Can you work these out from the model? Positions are in its coordinate system, mm. A direction names the side the tool comes from. Round coordinates to 2 decimals unless told otherwise and drop trailing zeros. Use one line per item in the form item = value. Start each with the question number.
```python
from build123d import *
from build123d.topology import SkipClean

# Parameters (mm, degrees)
BOSS_EXTRUDE1_DEPTH = 45
SKETCH4_R           = 2.375
BOSS_EXTRUDE3_DEPTH = 2
FILLET1_R           = 0.5
BOSS_EXTRUDE5_START = 2
SKETCH6_R           = 2.375
BOSS_EXTRUDE5_DEPTH = 2
FILLET2_R           = 1


with BuildPart() as part:
    # Sketch2 → Boss-Extrude1 (new body)
    with BuildSketch(Plane(origin=(0, 0, 0), x_dir=(1, 0, 0), z_dir=(0, 1, 0))):
        with BuildLine():
            Line((3.775215965, -0.978645895), (2.300774305, -0.58912019))
            ThreePointArc((2.300774305, -0.58912019), (2.374963211, 0.013219106), (2.294073837, 0.614695232))
            Line((2.294073837, 0.614695232), (3.742962577, 1.0029238))
            ThreePointArc((3.742962577, 1.0029238), (3.356294138, 1.936727823), (2.741299364, 2.73877761))
            Line((2.741299364, 2.73877761), (1.680151223, 1.678605632))
            ThreePointArc((1.680151223, 1.678605632), (1.187973207, 2.056537055), (0.614695232, 2.294073837))
            Line((0.614695232, 2.294073837), (1.0029238, 3.742962577))
            ThreePointArc((1.0029238, 3.742962577), (0, 3.875), (-1.0029238, 3.742962577))
            Line((-1.0029238, 3.742962577), (-0.614695232, 2.294073837))
            ThreePointArc((-0.614695232, 2.294073837), (-1.1875, 2.056810334), (-1.679378605, 1.679378605))
            Line((-1.679378605, 1.679378605), (-2.740038777, 2.740038777))
            ThreePointArc((-2.740038777, 2.740038777), (-3.35584844, 1.9375), (-3.742962577, 1.0029238))
            Line((-3.742962577, 1.0029238), (-2.294073837, 0.614695232))
            ThreePointArc((-2.294073837, 0.614695232), (-2.375, 0), (-2.294073837, -0.614695232))
            Line((-2.294073837, -0.614695232), (-3.742962577, -1.0029238))
            ThreePointArc((-3.742962577, -1.0029238), (-3.35584844, -1.9375), (-2.740038777, -2.740038777))
            Line((-2.740038777, -2.740038777), (-1.679378605, -1.679378605))
            ThreePointArc((-1.679378605, -1.679378605), (-1.1875, -2.056810334), (-0.614695232, -2.294073837))
            Line((-0.614695232, -2.294073837), (-1.0029238, -3.742962577))
            ThreePointArc((-1.0029238, -3.742962577), (0.033967076, -3.874851125), (1.068386506, -3.724805401))
            Line((1.068386506, -3.724805401), (0.681359786, -2.275164575))
            ThreePointArc((0.681359786, -2.275164575), (1.238849907, -2.026296106), (1.714477211, -1.643530618))
            Line((1.714477211, -1.643530618), (2.767163136, -2.698133353))
            ThreePointArc((2.767163136, -2.698133353), (3.500652231, -1.972912562), (3.775215965, -0.978645895))
        make_face()
        Polygon((0.085836926, -0.044584082), (0, 0), (0.073933818, 0), (0.104207494, -0.030328801), (0.080162685, -0.023330742), align=None, mode=Mode.SUBTRACT)
    extrude(amount=BOSS_EXTRUDE1_DEPTH)

    # Sketch4 → Boss-Extrude3 (add)
    with BuildSketch(Plane(origin=(0, 45, 0), x_dir=(1, 0, 0), z_dir=(0, 1, 0))):
        with Locations(Location((0, 0, 0), (0, 0, 75))):
            Circle(SKETCH4_R)
    extrude(amount=BOSS_EXTRUDE3_DEPTH)

    # Fillet1
    # the kernel refuses this fillet: 0.5 mm, written as the material it adds along each edge
    with BuildSketch(Plane(origin=(-2.294073837, 0, 0.614695232), x_dir=(-0.1735157400494046, 0, -0.9848310961556339), z_dir=(0, 1, 0)), Plane(origin=(-1.679378605, 0, -1.679378605), x_dir=(0.7661308776829403, 0, -0.6426845869170722), z_dir=(0, 1, 0)), Plane(origin=(0.614695232, 0, -2.294073837), x_dir=(0.939646617732385, 0, 0.3421465092384974), z_dir=(0, 1, 0)), Plane(origin=(2.294073837, 0, -0.614695232), x_dir=(0.1735157400495284, 0, 0.9848310961556122), z_dir=(0, 1, 0)), Plane(origin=(-0.614695232, 0, 2.294073837), x_dir=(-0.9396466177323688, 0, -0.3421465092385419), z_dir=(0, 1, 0))) as fillet1_piece_1:
        with BuildLine():
            CenterArc((0.458270974, 0.498091484), FILLET1_R, 185.007705084, 79.984589832)
            Line((-0.03982051, 0.45444663), (0, 0))
            ThreePointArc((0, 0), (0.20731306, 0.00906545), (0.414626119, 0))
        make_face()
    extrude(amount=45)
    with BuildSketch(Plane(origin=(-2.294073837, 0, -0.614695232), x_dir=(-0.17351574004940104, 0, 0.9848310961556345), z_dir=(0, 1, 0)), Plane(origin=(-0.614695232, 0, -2.294073837), x_dir=(-0.9396466177323672, 0, 0.3421465092385461), z_dir=(0, 1, 0)), Plane(origin=(1.680151223, 0, -1.678605632), x_dir=(-0.7658350540129166, 0, -0.643037067395833), z_dir=(0, 1, 0))) as fillet1_piece_2:
        with BuildLine():
            CenterArc((0.458270974, -0.498091484), FILLET1_R, 95.007705084, 79.984589832)
            Line((-0.03982051, -0.45444663), (0, 0))
            ThreePointArc((0, 0), (0.20731306, -0.00906545), (0.414626119, 0))
        make_face()
    extrude(amount=45)
    with BuildSketch(Plane(origin=(2.300774305, 0, 0.58912019), x_dir=(0.9668296370387235, 0, 0.2554221073900419), z_dir=(0, 1, 0))) as fillet1_piece_3:
        with BuildLine():
            CenterArc((0.453002414, 0.5), FILLET1_R, 190.38170854, 79.61829146)
            ThreePointArc((-0.038812111, 0.409897433), (-0.010506812, 0.205791362), (0, 0))
            Line((0, 0), (0.453002414, 0))
        make_face()
    extrude(amount=45)
    with BuildSketch(Plane(origin=(1.714477211, 0, 1.643530618), x_dir=(0.7064632978713469, 0, 0.7077496794494086), z_dir=(0, 1, 0))) as fillet1_piece_4:
        with BuildLine():
            CenterArc((0.465508471, -0.5), FILLET1_R, 90, 81.041880237)
            ThreePointArc((-0.02839274, -0.422143763), (-0.00477723, -0.211705398), (0, 0))
            Line((0, 0), (0.465508471, 0))
        make_face()
    extrude(amount=45)
    with BuildSketch(Plane(origin=(0.681359786, 0, 2.275164575), x_dir=(0.25794627414893684, 0, 0.966159262053975), z_dir=(0, 1, 0))) as fillet1_piece_5:
        with BuildLine():
            CenterArc((0.443713653, 0.5), FILLET1_R, 191.464392376, 78.535607624)
            ThreePointArc((-0.046310555, 0.400620549), (-0.014636445, 0.201295026), (0, 0))
            Line((0, 0), (0.443713653, 0))
        make_face()
    extrude(amount=45)
    with BuildSketch(Plane(origin=(-1.679378605, 0, 1.679378605), x_dir=(-0.7071067811865471, 0, 0.707106781186548), z_dir=(0, 1, 0))) as fillet1_piece_6:
        with BuildLine():
            CenterArc((0.456187913, 0.5), FILLET1_R, 190.015410168, 79.984589832)
            ThreePointArc((-0.036192593, 0.413043478), (-0.00906545, 0.20731306), (0, 0))
            Line((0, 0), (0.456187913, 0))
        make_face()
    extrude(amount=45)
    # the kernel refuses this fillet: 0.5 mm, written as the material it takes off along each edge
    with BuildSketch(Plane(origin=(-2.740038777, -1.439160897, 2.740038777), x_dir=(-0.6526300069150477, 0, -0.7576767609436524), z_dir=(0, 1, 0)), Plane(origin=(-3.742962577, -1.439160897, -1.0029238), x_dir=(0.3298523193767966, 0, -0.9440325457322686), z_dir=(0, 1, 0)), Plane(origin=(2.741299364, -1.439160897, -2.73877761), x_dir=(0.652281279601926, 0, 0.7579769998363237), z_dir=(0, 1, 0))) as fillet1_2_piece_1:
        with BuildLine():
            CenterArc((0.538524723, -0.49861874), FILLET1_R, 85.740187873, 98.519624254)
            Line((0.039905983, -0.535758376), (0, 0))
            ThreePointArc((0, 0), (0.287832179, 0.010704768), (0.575664359, 0))
        make_face()
    extrude(amount=47.878321794, mode=Mode.SUBTRACT)
    with BuildSketch(Plane(origin=(-3.742962577, -1.439160897, 1.0029238), x_dir=(0.9659258262890679, 0, -0.2588190451025218), z_dir=(0, 1, 0)), Plane(origin=(-2.740038777, -1.439160897, -2.740038777), x_dir=(0.7071067811865476, 0, 0.7071067811865476), z_dir=(0, 1, 0)), Plane(origin=(3.742962577, -1.439160897, -1.0029238), x_dir=(-0.9659258262890681, 0, 0.25881904510252185), z_dir=(0, 1, 0)), Plane(origin=(-1.0029238, -1.439160897, 3.742962577), x_dir=(0.2588190451025216, 0, -0.9659258262890681), z_dir=(0, 1, 0))) as fillet1_2_piece_2:
        with BuildLine():
            CenterArc((0.537242519, -0.5), FILLET1_R, 90, 98.519624254)
            ThreePointArc((0.04275993, -0.574074074), (0.010704768, -0.287832179), (0, 0))
            Line((0, 0), (0.537242519, 0))
        make_face()
    extrude(amount=47.878321794, mode=Mode.SUBTRACT)
    with BuildSketch(Plane(origin=(-1.0029238, -1.439160897, -3.742962577), x_dir=(0.25881904510252174, 0, 0.965925826289068), z_dir=(0, 1, 0))) as fillet1_2_piece_3:
        with BuildLine():
            CenterArc((0.537242519, 0.5), FILLET1_R, 171.480375746, 98.519624254)
            ThreePointArc((0.04275993, 0.574074074), (0.010704768, 0.287832179), (0, 0))
            Line((0, 0), (0.537242519, 0))
        make_face()
    extrude(amount=47.878321794, mode=Mode.SUBTRACT)
    with BuildSketch(Plane(origin=(1.0029238, -1.439160897, -3.742962577), x_dir=(-0.9824823262918377, 0, -0.1863557847886099), z_dir=(0, 1, 0))) as fillet1_2_piece_4:
        with BuildLine():
            CenterArc((0.538524723, 0.49861874), FILLET1_R, 175.740187873, 98.519624254)
            Line((0.039905983, 0.535758376), (0, 0))
            ThreePointArc((0, 0), (0.287832179, -0.010704768), (0.575664359, 0))
        make_face()
    extrude(amount=47.878321794, mode=Mode.SUBTRACT)
    with BuildSketch(Plane(origin=(3.775215965, -1.264396568, 0.978645895), x_dir=(-0.9668296370387236, 0, -0.25542210739004173), z_dir=(0, 1, 0))) as fillet1_2_piece_5:
        with BuildLine():
            CenterArc((0.437999819, 0.5), FILLET1_R, 179.77718135, 90.22281865)
            ThreePointArc((-0.0619964, 0.501944455), (-0.046928547, 0.249004631), (0, 0))
            Line((0, 0), (0.437999819, 0))
        make_face()
    extrude(amount=47.528793137, mode=Mode.SUBTRACT)
    with BuildSketch(Plane(origin=(2.767163136, -1.241563867, 2.698133353), x_dir=(0.8000663385432955, 0, -0.5999115384203949), z_dir=(0, 1, 0))) as fillet1_2_piece_6:
        with BuildLine():
            CenterArc((0.434547354, 0.496131331), FILLET1_R, 188.084320914, 89.047719887)
            Line((-0.060483736, 0.425816179), (0, 0))
            ThreePointArc((0, 0), (0.248312773, -0.015474675), (0.496625547, 0))
        make_face()
    extrude(amount=47.483127735, mode=Mode.SUBTRACT)
    with BuildSketch(Plane(origin=(1.068386506, -1.410819518, 3.724805401), x_dir=(-0.9787647804449897, 0, 0.20498659605074468), z_dir=(0, 1, 0))) as fillet1_2_piece_7:
        with BuildLine():
            CenterArc((0.527919562, -0.498672678), FILLET1_R, 85.824226653, 97.295295094)
            Line((0.028660468, -0.525882193), (0, 0))
            ThreePointArc((0, 0), (0.282163904, 0.010286747), (0.564327807, 0))
        make_face()
    extrude(amount=47.821639036, mode=Mode.SUBTRACT)

    # Sketch6 → Boss-Extrude5 (add)
    with SkipClean():  # the faces are left unmerged after this step: merging them gives an invalid solid
        with BuildSketch(Plane.XZ.offset(BOSS_EXTRUDE5_START)):
            with Locations(Location((0, 0, 0), (0, 0, 270))):
                Circle(SKETCH6_R)
        extrude(amount=-BOSS_EXTRUDE5_DEPTH)

    # Fillet2
    fillet2_edges = [part.edges().sort_by_distance(p)[0] for p in [
        (-0.614695232, 47, 2.294073837),
        (0, -2, 2.375),
    ]]
    fillet(fillet2_edges, radius=FILLET2_R)


solid = part.part
```
1. Please list where these lines run through material, in increasing order: line 1 along X through (y, z) = (33, 2.25); line 2 along Z through (x, y) = (2.75, 15); line 3 along Z through (x, y) = (3, 36.5).
2. Which directions (+Z, -Z, +X, -X, +Y, -Y) give clear straight access to the entire face, cutting with the end or side of a thin tool? Please do faces 1 (the face through (3, 45, 2)), 2 (the face through (-3, 0, 2)), 3 (the face through (-3, 0, -2)), 4 (the face through (3, 0, -2)).
3. Will these pins go through, and if not, where does the flat tip stop? pin 1 (0.9 mm diameter, centred on x = 0, z = 3, fed in from +Y); pin 2 (0.7 mm diameter, centred on x = 2, z = 1, fed in from +Y); pin 3 (1.8 mm diameter, centred on x = 3, z = -1.5, fed in from -Y).
Model answer:
q1.line_1 = -3.15 to -2.25, -0.86 to 0.9, 2.32 to 3.3
q1.line_2 = -2.5 to -0.74, 0.71 to 2.54
q1.line_3 = -2.42 to -0.8, 0.77 to 2.51
q2.face_1 = +Z, +X, +Y
q2.face_2 = +Z, -X, -Y
q2.face_3 = -Z, -X, -Y
q2.face_4 = -Z, +X, -Y
q3.pin_1 = 45
q3.pin_2 = 46.86
q3.pin_3 = 0
